from build123d import *

# Parameters (mm, degrees)
LOFTED_BENDS1_DEPTH     = 30
CUT_EXTRUDE1_DEPTH      = 291.9106392
CUT_EXTRUDE1_DEPTH_BACK = 291.9106392
SKETCH9_R               = 2


# Read off the part's stored shape, not the designer's step: Lofted Bends1
with BuildPart() as part:
    # Lofted Bends1 outline → Lofted Bends1 (new body)
    with BuildSketch(Plane.XY):
        with BuildLine():
            Line((-130, -110.629947141), (-130, -127))
            Line((-130, -127), (-128, -127))
            Line((-128, -127), (-128, -110.629947141))
            ThreePointArc((-128, -110.629947141), (-127.989562576, -110.506385525), (-127.958546096, -110.386325578))
            Line((-127.958546096, -110.386325578), (-125.853702275, -104.380395942))
            ThreePointArc((-125.853702275, -104.380395942), (-125.802985728, -104.267240099), (-125.734006394, -104.164195136))
            Line((-125.734006394, -104.164195136), (-45.607324148, -3.888698057))
            ThreePointArc((-45.607324148, -3.888698057), (-45.490716401, -3.772288571), (-45.351149992, -3.684711448))
            Line((-45.351149992, -3.684711448), (-37.841582221, -0.072791023))
            ThreePointArc((-37.841582221, -0.072791023), (-37.686040501, -0.018428275), (-37.522306162, 0))
            Line((-37.522306162, 0), (37.522306162, 0))
            ThreePointArc((37.522306162, 0), (37.686040501, -0.018428275), (37.841582221, -0.072791023))
            Line((37.841582221, -0.072791023), (45.351149992, -3.684711448))
            ThreePointArc((45.351149992, -3.684711448), (45.490716401, -3.772288571), (45.607324148, -3.888698057))
            Line((45.607324148, -3.888698057), (125.734006394, -104.164195136))
            ThreePointArc((125.734006394, -104.164195136), (125.802985728, -104.267240099), (125.853702275, -104.380395942))
            Line((125.853702275, -104.380395942), (127.958546096, -110.386325578))
            ThreePointArc((127.958546096, -110.386325578), (127.989562576, -110.506385525), (128, -110.629947141))
            Line((128, -110.629947141), (128, -127))
            Line((128, -127), (130, -127))
            Line((130, -127), (130, -110.629947141))
            ThreePointArc((130, -110.629947141), (129.961223114, -110.170893762), (129.845991373, -109.724849709))
            Line((129.845991373, -109.724849709), (127.741147552, -103.718920072))
            ThreePointArc((127.741147552, -103.718920072), (127.55272656, -103.298525993), (127.296456068, -102.91569563))
            Line((127.296456068, -102.91569563), (47.169773822, -2.640198551))
            ThreePointArc((47.169773822, -2.640198551), (46.736555305, -2.207716608), (46.218041274, -1.88235202))
            Line((46.218041274, -1.88235202), (38.708473503, 1.729568405))
            ThreePointArc((38.708473503, 1.729568405), (38.13060835, 1.93153568), (37.522306162, 2))
            Line((37.522306162, 2), (-37.522306162, 2))
            ThreePointArc((-37.522306162, 2), (-38.13060835, 1.93153568), (-38.708473503, 1.729568405))
            Line((-38.708473503, 1.729568405), (-46.218041274, -1.88235202))
            ThreePointArc((-46.218041274, -1.88235202), (-46.736555305, -2.207716608), (-47.169773822, -2.640198551))
            Line((-47.169773822, -2.640198551), (-127.296456068, -102.91569563))
            ThreePointArc((-127.296456068, -102.91569563), (-127.55272656, -103.298525993), (-127.741147552, -103.718920072))
            Line((-127.741147552, -103.718920072), (-129.845991373, -109.724849709))
            ThreePointArc((-129.845991373, -109.724849709), (-129.961223114, -110.170893762), (-130, -110.629947141))
        make_face()
    extrude(amount=LOFTED_BENDS1_DEPTH)

    # Sketch9 → Cut-Extrude1 (cut, two sides: drawn at the far end of the back side and taken through both)
    with BuildSketch(Plane(origin=(130, 0, 0), x_dir=(0, 0, -1), z_dir=(1, 0, 0)).offset(-CUT_EXTRUDE1_DEPTH_BACK)):
        with Locations(Location((-15, -118.814973571, 0), (0, 0, 90))):
            Circle(SKETCH9_R)
    extrude(amount=CUT_EXTRUDE1_DEPTH + CUT_EXTRUDE1_DEPTH_BACK, mode=Mode.SUBTRACT)


solid = part.part
Input: part model. Units: mm. Frame: model coordinates. A direction names the side the tool comes from. Give positions to 0.01 mm unless a question says otherwise; leave off trailing zeros. Loops run counter-clockwise (first coordinate to the right, second up) from the corner with the lowest first, then second, coordinate; pieces in that order, holes last. Notation, with made-up numbers: (44, -4.5) -> (101, -4.5) arc R15 cw to (101, 6.5) -> close; hole circle Ø2 at (57, -31). An arc over 180 degrees is marked (long way). Answer as a JSON object with one key per item and string values. Group by question number.
Item 1: Cut plane A-A, the plane y = -91.5. Return the cut outline in (x, z), and give its area (3 significant figures).
Item 2: Cut plane B-B, the plane x = 65. Return the cut outline in (y, z).
Item 3: Pin query (flat end, axial travel): P1, Ø2, axis at x = 55.5, z = 15.5, coming from the +Y side; P2, Ø1.5, axis at y = -30.5, z = 18.5, coming from the +X side; P3, Ø15, axis at x = 16.5, z = 17.5, coming from the -Y side. Return the tip coordinate at first contact, or that it passes through.
Item 4: Reachability of faces 4 (the flat face through (42.516, -0.102, 14.79)), 5 (the flat face through (-126.921, -107.425, 14.79)) from +Z, -Z, +X, -X, +Y, -Y: full face, straight path, thin tool, end or side. Return the list, or none.
Item 5: Pull-direction query (X, two-part tool) for faces 1 (the flat face through (-1, 0, 15)), 2 (the flat face through (130, -119, 11)), 3 (the flat face through (-130, -119, 11)); classes: released by +X, released by -X, zero draft, split by the parting line, or undercut.
Item 6: Line query: probe 1 along Y at (x, z) = (-9.5, 27.75); probe 2 along X at (y, z) = (-120.5, 22.75); probe 3 along X at (y, z) = (-53, 9.5). Output: solid intervals per line, ascending.
Checks:
{
 "1": {"outline": "(-118.17, 0) -> (-115.61, 0) -> (-115.61, 30) -> (-118.17, 30) -> close; (115.61, 0) -> (118.17, 0) -> (118.17, 30) -> (115.61, 30) -> close", "area": "154 mm²"},
 "2": {"outline": "(-28.16, 0) -> (-24.95, 0) -> (-24.95, 30) -> (-28.16, 30) -> close"},
 "3": {"P1": "stops at y = -11.81", "P2": "stops at x = 70.03", "P3": "stops at y = 0"},
 "4": {"face 4": "+Z, -Z, +X, +Y", "face 5": "+Z, -Z, -Y"},
 "5": {"face 1": "undercut", "face 2": "released by +X", "face 3": "released by -X"},
 "6": {"probe 1": "y = 0 to 2", "probe 2": "x = -130 to -128, 128 to 130", "probe 3": "x = -87.41 to -84.85, 84.85 to 87.41"}
}
